from build123d import *

# Parameters (mm, degrees)
F1_DEPTH   = 88.9
F1_FACE1_W = 26.3025612107
F1_FACE1_H = 88.9
F3_DEPTH   = 63.5
F5_DEPTH   = 3


# Not quite as in the source:
# - a feature names something its author has since deleted; it is built from what else it names


with BuildPart() as f1:
    # F0 (on Top) → F1 (new body)
    with BuildSketch(Plane.XY):
        Polygon((13.1512806053, 31.75), (-13.1512806053, 31.75), (-31.75, 13.1512806053), (-31.75, -13.1512806053), (-13.1512806053, -31.75), (13.1512806053, -31.75), (31.75, -13.1512806053), (31.75, 13.1512806053), align=None)
    extrude(amount=-F1_DEPTH)

    # F2 (on face) + F1_face1 (on face) → F3 (cut, through all)
    with BuildSketch(Plane(origin=(-31.75, 0, 0), x_dir=(0, -1, 0), z_dir=(-1, 0, 0))):
        Polygon((-19.05, -88.9), (-31.75, 0), (-31.75, -88.9), align=None)
        Polygon((31.75, -88.9), (31.75, 0), (13.1512806053, -36.823585695), (13.1512806053, -88.9), (14.6601814777, -88.9), align=None)
        Polygon((13.1512806053, -36.823585695), (-13.1512806053, -88.9), (-12.7, -88.9), (-6.35, -88.9), (0, -88.9), (8.3101814777, -88.9), (13.1512806053, -88.9), align=None)
    with BuildSketch(Plane(origin=(22.4506403027, -22.4506403027, -44.45), x_dir=(0.7071067812, 0.7071067812, 0), z_dir=(0.7071067812, -0.7071067812, 0))):
        Rectangle(F1_FACE1_W, F1_FACE1_H)
    extrude(amount=-F3_DEPTH, dir=(-1, 0, 0), mode=Mode.SUBTRACT)

    # F4 (on face) → F5 (join)
    with BuildSketch(Plane.XY):
        Polygon((13.1512806053, 31.75), (-13.1512806053, 31.75), (-31.75, 13.1512806053), (-31.75, -13.1512806053), (-13.1512806053, -31.75), (13.1512806053, -31.75), (31.75, -13.1512806053), (31.75, 13.1512806053), align=None)
        Polygon((-28.75, 10.7754608616), (-28.75, 11.9086399182), (-11.9086399182, 28.75), (11.9086399182, 28.75), (28.75, 11.9086399182), (28.75, 10.7754608616), (28.75, -10.7754608616), (28.75, -11.9086399182), (11.9086399182, -28.75), (-11.9086399182, -28.75), (-28.75, -11.9086399182), (-28.75, -10.7754608616), align=None, mode=Mode.SUBTRACT)
        with BuildLine():
            add(Edge.make_bspline(
                [(4.8083327711, 10.5354869738), (5.9249649259, 10.4834162819), (7.339599469, 10.0059956165), (8.3643975774, 9.1943899894), (8.5739761095, 8.9890481737)],
                knots=[0, 0, 0, 0, 0.0796423572, 0.1022272486, 0.1022272486, 0.1022272486, 0.1022272486], degree=3))
            add(Edge.make_bspline(
                [(4.8083327711, 10.5354869738), (3.6917006162, 10.4834162819), (2.2770660731, 10.0059956165), (1.2522679647, 9.1943899894), (1.0426894326, 8.9890481737)],
                knots=[0, 0, 0, 0, 0.0796423572, 0.1022272486, 0.1022272486, 0.1022272486, 0.1022272486], degree=3))
            add(Edge.make_bspline(
                [(-0.5542273499, -6.0097523046), (-0.6853048791, -5.4911473404), (-1.2029837025, -2.5307480598), (-1.3645767848, 4.0861219904), (0.1727738224, 7.9642019091), (1.0426894326, 8.9890481737)],
                knots=[0.6521796741, 0.6521796741, 0.6521796741, 0.6521796741, 0.683293281, 0.8153772216, 0.9015400151, 0.9015400151, 0.9015400151, 0.9015400151], degree=3))
            add(Edge.make_bspline(
                [(-0.5542273499, -6.0097523046), (-0.1219359708, -7.2774050993), (0.4855176774, -8.258165167), (1.158925978, -8.9826247772)],
                knots=[0.3319618275, 0.3319618275, 0.3319618275, 0.3319618275, 0.3946519049, 0.3946519049, 0.3946519049, 0.3946519049], degree=3))
            add(Edge.make_bspline(
                [(4.8083327711, -10.5354869738), (3.6099604652, -10.4237469099), (2.1738291685, -9.8473995471), (1.158925978, -8.9826247772)],
                knots=[0.4948947439, 0.4948947439, 0.4948947439, 0.4948947439, 0.5783031472, 0.5783031472, 0.5783031472, 0.5783031472], degree=3))
            add(Edge.make_bspline(
                [(4.8083327711, -10.5354869738), (6.0067050769, -10.4237469099), (7.4428363737, -9.8473995471), (8.4577395641, -8.9826247772)],
                knots=[0.4948947439, 0.4948947439, 0.4948947439, 0.4948947439, 0.5783031472, 0.5783031472, 0.5783031472, 0.5783031472], degree=3))
            add(Edge.make_bspline(
                [(10.170892892, -6.0097523046), (9.7386015129, -7.2774050993), (9.1311478647, -8.258165167), (8.4577395641, -8.9826247772)],
                knots=[0.3319618275, 0.3319618275, 0.3319618275, 0.3319618275, 0.3946519049, 0.3946519049, 0.3946519049, 0.3946519049], degree=3))
            add(Edge.make_bspline(
                [(10.170892892, -6.0097523046), (10.3019704212, -5.4911473404), (10.8196492446, -2.5307480598), (10.9812423269, 4.0861219904), (9.4438917197, 7.9642019091), (8.5739761095, 8.9890481737)],
                knots=[0.6521796741, 0.6521796741, 0.6521796741, 0.6521796741, 0.683293281, 0.8153772216, 0.9015400151, 0.9015400151, 0.9015400151, 0.9015400151], degree=3))
        make_face()
        with BuildLine():
            add(Edge.make_bspline(
                [(4.8083327711, 7.7876993455), (3.9534414496, 7.4218723248), (2.0820207972, 6.6210497822), (1.660966503, 2.272494011), (1.6738338819, 0)],
                knots=[0, 0, 0, 0, 0.2110894815, 0.4620905666, 0.4620905666, 0.4620905666, 0.4620905666], degree=3))
            add(Edge.make_bspline(
                [(4.8083327711, 7.7876993455), (5.6632240926, 7.4218723248), (8.028214212, 6.4098404237), (8.0974839635, -3.0892679636), (6.9910117402, -7.135194286), (5.4397234852, -7.47767614), (4.8083327711, -7.617069874)],
                knots=[0, 0, 0, 0, 0.2110894815, 0.5839625756, 0.8306683715, 1, 1, 1, 1], degree=3))
            add(Edge.make_bspline(
                [(1.6738338819, 0), (1.6800815574, -1.1033952726), (1.8712186248, -4.3765266238), (2.6256538019, -7.135194286), (4.1769420569, -7.47767614), (4.8083327711, -7.617069874)],
                knots=[0.4620905666, 0.4620905666, 0.4620905666, 0.4620905666, 0.5839625756, 0.8306683715, 1, 1, 1, 1], degree=3))
        make_face(mode=Mode.SUBTRACT)
        with BuildLine():
            Line((20.6052474678, 10.1401684806), (13.9625072479, 10.1401684806))
            Line((13.9625072479, 10.1401684806), (13.9625072479, -10.1387687027))
            Line((13.9625072479, -10.1387687027), (16.9827528298, -10.1387687027))
            Line((16.9827528298, -10.1387687027), (16.9827528298, -1.2698972132))
            Line((16.9827528298, -1.2698972132), (20.6052474678, -1.2698972132))
            add(Edge.make_bspline(
                [(20.6052474678, 10.1401684806), (21.8779731079, 9.8412745125), (24.3142685907, 9.2691213309), (25.4822457744, 6.1351724103), (25.736421693, 2.6562033682), (24.2123159942, -0.1800935194), (21.4538469207, -1.3948664952), (20.8225355964, -1.3018962221), (20.6052474678, -1.2698972132)],
                knots=[0, 0, 0, 0, 0.1937641782, 0.3709100981, 0.5596905933, 0.7399766879, 0.9105037773, 1, 1, 1, 1], degree=3))
        make_face()
        with BuildLine():
            Line((20.2160011977, 1.5110635431), (16.9827528298, 1.5110635431))
            Line((16.9827528298, 1.5110635431), (16.9827528298, 7.4263564311))
            Line((16.9827528298, 7.4263564311), (20.2160011977, 7.4263564311))
            add(Edge.make_bspline(
                [(20.2160011977, 7.4263564311), (21.1544893682, 7.4114310555), (22.7486394765, 6.0097179724), (22.8736105917, 3.1708769977), (21.149745211, 1.4233636903), (20.2160011977, 1.5110635431)],
                knots=[0, 0, 0, 0, 0.3295814167, 0.6602854532, 1, 1, 1, 1], degree=3))
        make_face(mode=Mode.SUBTRACT)
        with BuildLine():
            ThreePointArc((-16.8338958174, -4.1077076457), (-19.6410734206, -7.564034438), (-22.4482510239, -4.1077076457))
            Line((-22.4482510239, -4.1077076457), (-25.4293251783, -4.1077076457))
            ThreePointArc((-25.4293251783, -4.1077076457), (-18.1588622297, -10.3219857216), (-14.8939756829, -1.3321359272))
            add(Edge.make_bspline(
                [(-15.8727969974, 0), (-15.4709741473, -0.3938739537), (-15.0835029781, -0.853099511), (-14.8939756829, -1.3321359272)],
                knots=[0, 0, 0, 0, 1.6530811518, 1.6530811518, 1.6530811518, 1.6530811518], degree=3))
            add(Edge.make_bspline(
                [(-21.5829703957, 5.279887002), (-21.6180322262, 4.9093177243), (-21.7144690872, 3.8900743649), (-18.3106174987, 2.2689761454), (-16.6874966749, 0.7582732743), (-15.8727969974, 0)],
                knots=[0, 0, 0, 0, 0.221505784, 0.6092472123, 1, 1, 1, 1], degree=3))
            ThreePointArc((-21.5829703957, 5.279887002), (-19.2209649831, 7.6604824432), (-16.8589595705, 5.279887002))
            Line((-16.8589595705, 5.279887002), (-14.1183091328, 5.3153838962))
            ThreePointArc((-14.1183091328, 5.3153838962), (-19.22945472, 10.4010814839), (-24.3236490835, 5.298404446))
            add(Edge.make_bspline(
                [(-24.3236490835, 5.298404446), (-24.3557528234, 4.7439102233), (-24.4260352796, 3.5299950823), (-23.0471913533, 1.3752329572), (-21.5360686477, 0.4670374949), (-20.7589771599, 0)],
                knots=[0, 0, 0, 0, 0.2900044831, 0.6348863858, 1, 1, 1, 1], degree=3))
            add(Edge.make_bspline(
                [(-20.7589771599, 0), (-19.6156120227, -0.7838167648), (-18.2336909625, -1.7311719529), (-17.5404152252, -2.6957135463), (-17.4353591755, -2.8625837034)],
                knots=[0, 0, 0, 0, 0.5794694701, 0.7003721194, 0.7003721194, 0.7003721194, 0.7003721194], degree=3))
            ThreePointArc((-17.4353591755, -2.8625837034), (-17.0584672604, -3.448356091), (-16.8338958174, -4.1077076457))
        make_face()
        Polygon((-9.3714222312, 7.4263564311), (-9.3714222312, -10.1387687027), (-6.427643355, -10.1387687027), (-6.427643355, 7.4263564311), (-2.6484197006, 7.4263564311), (-2.6484197006, 10.1401684806), (-6.427643355, 10.1401684806), (-9.3714222312, 10.1401684806), (-13.0321141332, 10.1401684806), (-13.0321141332, 7.4263564311), align=None)
        with BuildLine():
            add(Edge.make_bspline(
                [(-0.5542273499, -6.0097523046), (-0.6853048791, -5.4911473404), (-1.2029837025, -2.5307480598), (-1.3645767848, 4.0861219904), (0.1727738224, 7.9642019091), (1.0426894326, 8.9890481737)],
                knots=[0.6521796741, 0.6521796741, 0.6521796741, 0.6521796741, 0.683293281, 0.8153772216, 0.9015400151, 0.9015400151, 0.9015400151, 0.9015400151], degree=3))
            add(Edge.make_bspline(
                [(1.0426894326, 8.9890481737), (0.4633846395, 8.4214542659), (-1.0609269861, 5.8291860693), (-1.6974790085, -2.0230291515), (-0.6825603591, -5.6334281267), (-0.5542273499, -6.0097523046)],
                knots=[0.1022272486, 0.1022272486, 0.1022272486, 0.1022272486, 0.1646550922, 0.3133512175, 0.3319618275, 0.3319618275, 0.3319618275, 0.3319618275], degree=3))
        make_face()
        with BuildLine():
            add(Edge.make_bspline(
                [(8.5739761095, 8.9890481737), (9.1532809026, 8.4214542659), (10.6775925282, 5.8291860693), (11.3141445506, -2.0230291515), (10.2992259012, -5.6334281267), (10.170892892, -6.0097523046)],
                knots=[0.1022272486, 0.1022272486, 0.1022272486, 0.1022272486, 0.1646550922, 0.3133512175, 0.3319618275, 0.3319618275, 0.3319618275, 0.3319618275], degree=3))
            add(Edge.make_bspline(
                [(10.170892892, -6.0097523046), (10.3019704212, -5.4911473404), (10.8196492446, -2.5307480598), (10.9812423269, 4.0861219904), (9.4438917197, 7.9642019091), (8.5739761095, 8.9890481737)],
                knots=[0.6521796741, 0.6521796741, 0.6521796741, 0.6521796741, 0.683293281, 0.8153772216, 0.9015400151, 0.9015400151, 0.9015400151, 0.9015400151], degree=3))
        make_face()
        with BuildLine():
            add(Edge.make_bspline(
                [(4.8083327711, -10.5354869738), (3.6099604652, -10.4237469099), (2.1738291685, -9.8473995471), (1.158925978, -8.9826247772)],
                knots=[0.4948947439, 0.4948947439, 0.4948947439, 0.4948947439, 0.5783031472, 0.5783031472, 0.5783031472, 0.5783031472], degree=3))
            add(Edge.make_bspline(
                [(1.158925978, -8.9826247772), (1.4164965069, -9.2597218145), (2.5336297837, -10.2613938856), (3.712598623, -10.6376567279), (4.8083327711, -10.5354869738)],
                knots=[0.3946519049, 0.3946519049, 0.3946519049, 0.3946519049, 0.4186301011, 0.4948947439, 0.4948947439, 0.4948947439, 0.4948947439], degree=3))
        make_face()
        with BuildLine():
            add(Edge.make_bspline(
                [(8.4577395641, -8.9826247772), (8.2001690352, -9.2597218145), (7.0830357584, -10.2613938856), (5.9040669191, -10.6376567279), (4.8083327711, -10.5354869738)],
                knots=[0.3946519049, 0.3946519049, 0.3946519049, 0.3946519049, 0.4186301011, 0.4948947439, 0.4948947439, 0.4948947439, 0.4948947439], degree=3))
            add(Edge.make_bspline(
                [(4.8083327711, -10.5354869738), (6.0067050769, -10.4237469099), (7.4428363737, -9.8473995471), (8.4577395641, -8.9826247772)],
                knots=[0.4948947439, 0.4948947439, 0.4948947439, 0.4948947439, 0.5783031472, 0.5783031472, 0.5783031472, 0.5783031472], degree=3))
        make_face()
    extrude(amount=F5_DEPTH)


solid = f1.part
Could you check a few things on this model? Use its own coordinates, in mm. A direction names the side the tool comes from. Give positions to 0.01 mm unless a question says otherwise; leave off trailing zeros. Order: outer loops, then holes, each group sorted by start corner. A loop starts at its lowest first (then second) coordinate and runs counter-clockwise, first axis right, second up.
Item 1: I'm going to push flat-ended pins straight in: pin 1 (5 mm diameter, centred on y = 24.5, z = -52.5, fed in from -X); pin 2 (12 mm diameter, centred on x = 1.5, z = -64.5, fed in from -Y); pin 3 (5 mm diameter, centred on x = 8.5, z = -20.5, fed in from -Y). Where does each tip first touch, or does it pass through?
Item 2: I need wall thicknesses on line 1 (Z direction, x = 3, y = 14); line 2 (Z direction, x = -2, y = -17); line 3 (Y direction, x = -6, z = -69). Which ranges of each line are inside material? Lowest first, please.
Item 3: If we section it at D-D, the plane z = -42.5: Write out the boundary of the cut face in (x, y), plus the area to 3 significant figures.
Item 4: If we section it at C-C, the plane y = -21: Write out the boundary of the cut face in (x, z), plus the area to 3 significant figures.
Item 5: If we section it at B-B, the plane z = -27: Write out the boundary of the cut face in (x, y).
Item 6: If we mould it in two halves opening along Y, with no side actions, what happens to faces 3 (the face through (21, -21, 3)), 4 (the face through (16.983, 4, 1)), 5 (the face through (-24.6, -20.3, -12.8)), 6 (the face through (-0.36, 23.9, -54.95))? For each: pulls with the +Y half, pulls with the -Y half, needs draft (parallel to the pull), parting line crosses it, or undercut.
Item 7: If we section it at A-A, the plane x = -4.5: Write out the boundary of the cut face in (y, z), plus the area to 3 significant figures.
Item 8: For faces 1 (the face through (0, 16, -88.9)), 2 (the face through (-19.1, 10.4, 1.5)), which set-ups out of +Z, -Z, +X, -X, +Y, -Y let a thin tool reach every point of the face, with its end or its side?
Values:
1. pin 1: stops at x = -22.9
1. pin 2: stops at y = -2.2
1. pin 3: stops at y = -22.66
2. line 1: z = -88.9 to 0
2. line 2: z = -29.2 to 0
2. line 3: y = 3.1 to 21.89
3. outline: (-31.75, -10.28) - (31.75, -10.28) - (31.75, 13.15) - (19.22, 25.68) - (-19.22, 25.68) - (-31.75, 13.15) - close
3. area: 2,130 mm2
4. outline: (-23.9, -21.28) - (23.9, -21.28) - (23.9, 3) - (19.66, 3) - (19.66, 0) - (-19.66, 0) - (-19.66, 3) - (-23.9, 3) - close
4. area: 1,040 mm2
5. outline: (-31.75, -13.15) - (-26.79, -18.11) - (26.79, -18.11) - (31.75, -13.15) - (31.75, 13.15) - (17.01, 27.89) - (-17.01, 27.89) - (-31.75, 13.15) - close
6. face 3: needs draft
6. face 4: undercut
6. face 5: pulls with the -Y half
6. face 6: pulls with the +Y half
7. outline: (-31.75, 0) - (13.15, -88.9) - (19.05, -88.9) - (31.75, 0) - (31.75, 3) - (28.75, 3) - (28.75, 0) - (10.14, 0) - (10.14, 3) - (7.43, 3) - (7.43, 0) - (-28.75, 0) - (-28.75, 3) - (-31.75, 3) - close
7. area: 3,110 mm2
8. face 1: -Z, +X, -X, +Y, -Y
8. face 2: +Z
